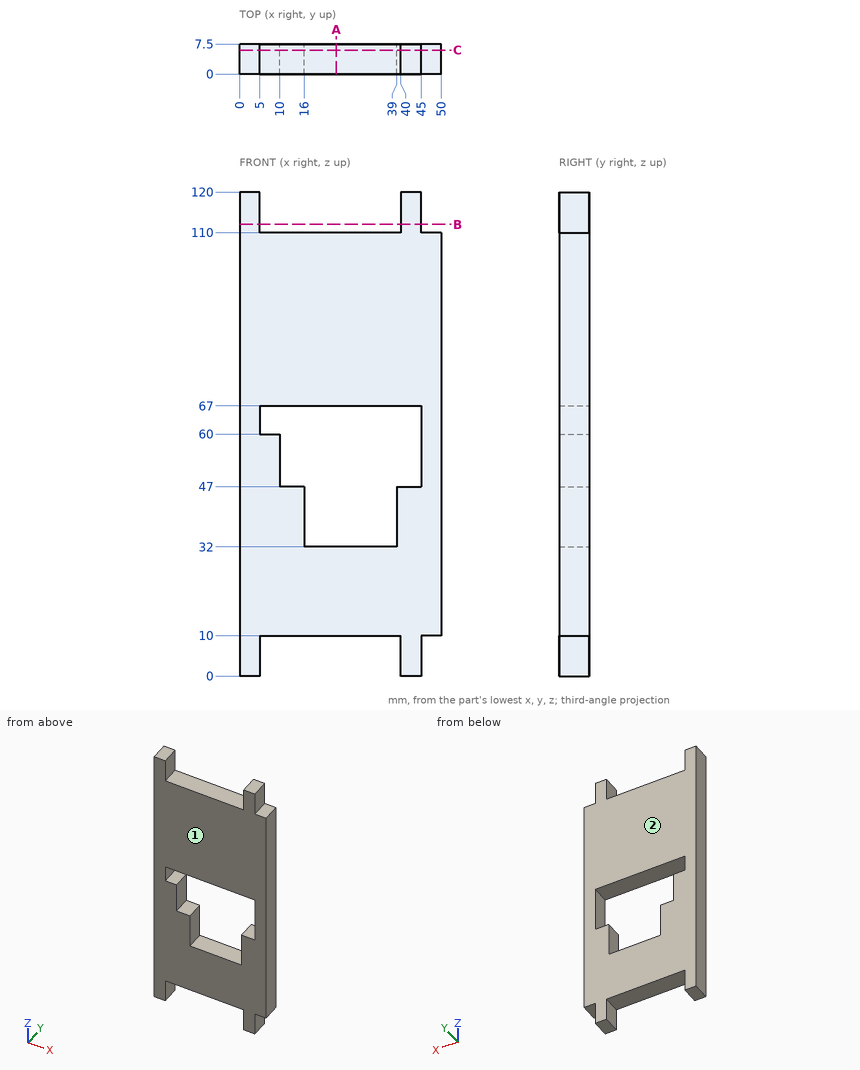
The drawing under review shows one solid part. Ordinate dimensions are in mm from its lowest x, y, z. Round coordinates to 2 decimals unless told otherwise and drop trailing zeros. Loops run counter-clockwise (first coordinate to the right, second up) from the corner with the lowest first, then second, coordinate; pieces in that order, holes last. Notation, with made-up numbers: (45, 19) - (51, 19) arc R32 cw to (51, 45) - close; hole circle Ø2 at (53, 68.25). An arc over 180 degrees is marked (long way). One line per question, with ' | ' between items.
Q1. For pin 1 (1.5 mm diameter, centred on x = 48, y = 2, fed in from -Z); pin 2 (1.8 mm diameter, centred on x = 12.5, y = 4, fed in from +Z), all flat-tipped, find the tip position at first contact; note any pin that passes through.
Taken from the geometry:
pin 1: stops at z = 10 | pin 2: stops at z = 110
Q2. The part is to be moulded in two halves that separate along Y. For the marked faces 1 and 2, say which applies: released by +Y, released by -Y, zero draft, split by the parting line, or undercut.
Taken from the geometry:
face 1: released by -Y | face 2: released by +Y
Q3. Take a section at C-C (y = 6). Give the boundary of the cut face in (x, z), and give its area (3 significant figures).
Taken from the geometry:
outline: (0, 0) - (5, 0) - (5, 10) - (40, 10) - (40, 0) - (45, 0) - (45, 10) - (50, 10) - (50, 110) - (45, 110) - (45, 120) - (40, 120) - (40, 110) - (5, 110) - (5, 120) - (0, 120) - close; hole (5, 60) - (10, 60) - (10, 47) - (16, 47) - (16, 32) - (39, 32) - (39, 47) - (45, 47) - (45, 67) - (5, 67) - close | area: 4,120 mm²
Q4. Take a section at B-B (z = 112). Give the boundary of the cut face in (x, y), and give its area (3 significant figures).
Taken from the geometry:
outline: (0, 0) - (5, 0) - (5, 7.5) - (0, 7.5) - close; (40, 0) - (45, 0) - (45, 7.5) - (40, 7.5) - close | area: 75.0 mm²
Q5. For line 1 along X through (y, z) = (6.5, 9); line 2 along Z through (x, y) = (11, 4.75); line 3 along X through (y, z) = (6.5, 59.5), list the stretches that pass through material, from the lowest coordinate up. Write a range as [from, to].
Taken from the geometry:
line 1: x = [0, 5], [40, 45] | line 2: z = [10, 47], [67, 110] | line 3: x = [0, 10], [45, 50]
Q6. Take a section at A-A (x = 24). Give the boundary of the cut face in (y, z).
Taken from the geometry:
outline: (0, 10) - (7.5, 10) - (7.5, 32) - (0, 32) - close; (0, 67) - (7.5, 67) - (7.5, 110) - (0, 110) - close
